Read the model definition and answer for the solid it produces. Units are mm, in the model's axes. Face numbers are marked on the shaded views. A direction names the side the tool comes from. Round coordinates to 2 decimals unless told otherwise and drop trailing zeros. Write each loop counter-clockwise with the first axis right and the second up, starting at its lowest first coordinate (ties: lowest second). Pieces come first, ordered by that corner, then holes. Notation, with made-up numbers: (-26, 88) - (13, 88) arc R16 cw to (13, 105) - close; hole circle Ø9 at (-8, 35). An arc over 180 degrees is marked (long way). Use one line per item in the form item = value. Start each with the question number.
1) The part is cut by section C-C, the plane y = 10.5. Give the vertices of the cut face in (x, z).
2) Each of these flat-tipped pins is pushed along its axis until it touches: pin 1 (4 mm diameter, centred on x = 1.5, y = 18, fed in from -Z); pin 2 (4 mm diameter, centred on y = 8, z = -4.5, fed in from +X); pin 3 (5 mm diameter, centred on y = 23.5, z = -2.5, fed in from -X). Where does it stop, or does it pass through?
3) Consider line 1 along Y through (x, z) = (-0.5, 0); line 2 along Z through (x, y) = (0, 27); line 3 along Y through (x, z) = (3.5, -1.5). Determine where each line is inside the solid, lowest interval first. Write a range as from..to.
4) The part is cut by section A-A, the plane z = 0. Give the vertices of the cut face in (x, y).
5) The part is cut by section B-B, the plane x = 0. Give the vertices of the cut face in (y, z), plus the area to 3 significant figures.
6) The part is cut by section D-D, the plane y = 26. Give the vertices of the cut face in (x, z).
7) For the marked faces 1 and 2, determine the directions among +Z, -Z, +X, -X, +Y, -Y from which every point of the face is accessible in a straight line to the end or side of a thin tool.
from build123d import *

# Parameters (mm, degrees)
CUT_EXTRUDE1_DEPTH      = 32.176914536
CUT_EXTRUDE1_DEPTH_BACK = 32.176914536
SKETCH3_R               = 1.5


with BuildPart() as part:
    # Sketch2 → Revolve2 (revolve)
    with BuildSketch(Plane.XY):
        Polygon((0, 0), (-6, 0), (-6, 2), (-4, 4), (-4, 5), (-3, 5), (-3, 30), (0, 30), align=None)
    revolve(axis=Axis((0, 30, 0), (0, -1, 0)))

    # Sketch3 → Cut-Extrude1 (cut, two sides: drawn at the far end of the back side and taken through both)
    with BuildSketch(Plane(origin=(0, 0, 0), x_dir=(0, 0, -1), z_dir=(1, 0, 0)).offset(-CUT_EXTRUDE1_DEPTH_BACK)):
        with Locations((0, 27)):
            Circle(SKETCH3_R)
    extrude(amount=CUT_EXTRUDE1_DEPTH + CUT_EXTRUDE1_DEPTH_BACK, mode=Mode.SUBTRACT)


solid = part.part
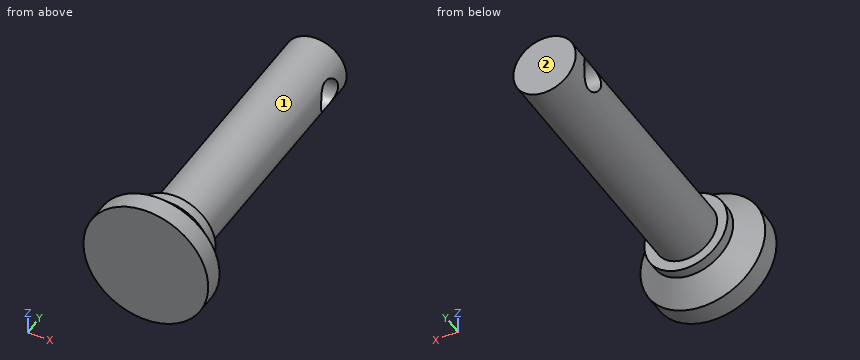
Geometry results:
q1.outline = circle Ø6 at (0, 0)
q2.pin_1 = -3
q2.pin_2 = 1.66
q2.pin_3 = -3
q3.line_1 = 0..25.5, 28.5..30
q3.line_2 = -3..-1.5, 1.5..3
q3.line_3 = 0..5
q4.outline = (-6, 0) - (6, 0) - (6, 2) - (4, 4) - (4, 5) - (3, 5) - (3, 25.5) - (-3, 25.5) - (-3, 5) - (-4, 5) - (-4, 4) - (-6, 2) - close; (-3, 28.5) - (3, 28.5) - (3, 30) - (-3, 30) - close
q5.outline = (0, -6) - (2, -6) - (4, -4) - (5, -4) - (5, -3) - (30, -3) - (30, 3) - (5, 3) - (5, 4) - (4, 4) - (2, 6) - (0, 6) - close; hole circle Ø3 at (27, 0)
q5.area = 195 mm2
q6.outline = (-2.78, -1.12) arc R3 ccw to (2.78, -1.12) - close; (-2.78, 1.12) - (2.78, 1.12) arc R3 ccw to start
q7.face_1 = +Y
q7.face_2 = +Z, -Z, +X, -X, +Y
